Autodesk Fusion 360 part; units mm, degrees
sketch "Sketch1" plane through (0, 0, 0) normal (0, 1, 0) x (1, 0, 0)
  line L0 (20, -20) -> (-20, -20)
  line L1 (-20, -20) -> (-20, 20)
  line L2 (-20, 20) -> (20, 20)
  line L3 (20, 20) -> (20, -20)
  line L4 (20, -20) -> (-20, 20) construction
  line L5 (-20, -20) -> (20, 20) construction
  line L6 (-20, 4) -> (-15, 4)
  line L7 (-15, 4) -> (-15, -4)
  line L8 (-15, -4) -> (-20, -4)
  line L9 (-20, -4) -> (-20, 4)
  line L10 (-4, 20) -> (4, 20)
  line L11 (4, 20) -> (4, 15)
  line L12 (4, 15) -> (-4, 15)
  line L13 (-4, 15) -> (-4, 20)
  line L14 (20, 4) -> (15, 4)
  line L15 (15, 4) -> (15, -4)
  line L16 (15, -4) -> (20, -4)
  line L17 (20, -4) -> (20, 4)
  line L18 (-4, -20) -> (4, -20)
  line L19 (4, -20) -> (4, -15)
  line L20 (4, -15) -> (-4, -15)
  line L21 (-4, -15) -> (-4, -20)
  dimension "d1" = 40
  dimension "d2" = 40
  dimension "d3" = 5
  dimension "d4" = 8
  dimension "d5" = 16
  dimension "d6" = 5
  dimension "d7" = 16
  dimension "d8" = 8
  dimension "d9" = 5
  dimension "d10" = 5
  dimension "d11" = 8
  dimension "d12" = 8
  dimension "d13" = 16
  dimension "d14" = 16
extrude "Extrude1" add sketch "Sketch1" against normal blind 3 contours L0 L1 L2 L3 L6 L7 L8 L11 L12 L13 L14 L15 L16 L19 L20 L21
extrude "Extrude2" add sketch "Sketch1" against normal blind 8 contours L0 L18 L19 L20 L21 | L3 L14 L15 L16 L17 | L1 L6 L7 L8 L9 | L2 L10 L11 L12 L13
hole "Hole1" at (0, 0, 0) direction (0, -1, 0) diameter 9 depth 30 tip angle 118
fillet "Fillet1" radius 4 4 edges at (20, -1.5, -20) (-20, -1.5, -20) (20, -1.5, 20) (-20, -1.5, 20)
sketch "Sketch2" plane through (0, 0, 0) normal (0, 1, 0) x (1, 0, 0)
  line L0 (21, 21) -> (-21, 21)
  line L1 (-21, 21) -> (-21, -21)
  line L2 (-21, -21) -> (21, -21)
  line L3 (21, -21) -> (21, 21)
  line L4 (21, 21) -> (-21, -21) construction
  line L5 (-21, 21) -> (21, -21) construction
  dimension "d24" = 42
  dimension "d25" = 42
extrude "Extrude3" add sketch "Sketch2" sketch "Sketch1" along normal blind 30 of sketch 2 contours L0 L1 L2 L3 L6 L7 L8 L11 L12 L13 L14 L15 L16 L19 L20 L21
sketch "Sketch3" plane through (0, 30, 0) normal (0, 1, 0) x (-1, 0, 0)
  line L0 (-21, 21) -> (-21, -21)
  line L1 (-21, -21) -> (21, -21)
  line L2 (21, -21) -> (21, 21)
  line L3 (21, 21) -> (-21, 21)
  circle A0 centre (41, 0) radius 7.5
  circle A1 centre (-41, 0) radius 7.5
  line L4 (-21, -21) -> (-44.9086, -6.401)
  line L5 (-21, 21) -> (-44.9086, 6.401)
  line L6 (21, 21) -> (44.9086, 6.401)
  line L7 (21, -21) -> (44.9086, -6.401)
  point P0 (41, 0)
  point P1 (-41, 0)
  dimension "d28" = 21
  dimension "d29" = 41
  dimension "d30" = 41
  dimension "d31" = 15
  dimension "d32" = 15
extrude "Extrude4" add sketch "Sketch3" against normal blind 5 contours L0 A1 L4 L5 | L2 A0 L6 L7 | A1 | A0
sketch "Sketch4" plane through (0, 0, 0) normal (0, -1, 0) x (1, 0, 0)
  circle A0 centre (0, 0) radius 4.5
  circle A1 centre (0, 0) radius 4.5
sketch "Sketch5" plane through (0, 0, 0) normal (0, 1, 0) x (-1, 0, 0)
sketch "Sketch6" plane through (0, 30, 0) normal (0, 1, 0) x (-1, 0, 0)
  circle A0 centre (0, 0) radius 4.5
hole "Hole2" at (0, 30, 0) direction (0, -1, 0) diameter 10 depth 90 tip angle 118 counterbore diameter 14 counterbore depth 26
hole "Hole3" at (-41, 30, 0) at (41, 30, 0) direction (0, -1, 0) diameter 4.234 depth 90 tip angle 118
fillet "Fillet2" radius 4 4 edges at (21, 12.5, -21) (-21, 12.5, -21) (-21, 12.5, 21) (21, 12.5, 21)
equation "d6 = d3"
equation "d7 = d5"
equation "d8 = d4"
equation "d9 = d3"
equation "d10 = d3"
equation "d11 = d4"
equation "d12 = d4"
equation "d13 = d7"
equation "d14 = d7"
Model file for the job. Use its own axes, mm. A direction names the side the tool comes from. Give positions to 0.01 mm unless a question says otherwise; leave off trailing zeros. Loops run counter-clockwise (first coordinate to the right, second up) from the corner with the lowest first, then second, coordinate; pieces in that order, holes last.
1) Flat gauge pins, fed straight in: pin 1 Ø5.5 at (y, z) = (-4.5, -17) entering from -X; pin 2 Ø9 at (y, z) = (-3, -4.5) entering from -X; pin 3 Ø5.5 at (x, y) = (-17, -5.5) entering from -Z. Where does each tip first touch, or does it go through?
2) Saw through at B-B (y = 15). Write the cut outline in (x, z), plus the area to 3 significant figures.
3) Saw through at A-A (z = 0). Count the separate pieces of the cut face and the enclosed holes in it, plus the area to 3 significant figures.
4) Saw through at D-D (y = -5). Write the cut outline in (x, z), plus the area to 3 significant figures.
5) Saw through at C-C (x = 0). Write the cut outline in (y, z), plus the area to 3 significant figures.
6) Wall check: line 1 (X direction, y = 26.8, z = 0); line 2 (X direction, y = 9.75, z = 0); line 3 (Y direction, x = 2, z = 9). Give the ranges that are in metal, low to high.
7) Pull direction X, two halves, no side cores. Call faces 1 (the flat face through (-18, -8, 0)), 2 (the flat face through (-20, -3, 0)), 3 (the flat face through (-5, 4, -2)): +X half, -X half, draft (parallel to the pull), parting line (faces both ways), or undercut.
8) Tool access for faces 4 (the cylindrical face through (2.681, 16.818, 6.466)), 5 (the cylindrical face through (18.859, -1.521, 18.797)), 6 (the flat face through (-17, -5, 4)), 7 (the flat face through (21, 12, 0)): list every direction of +Z, -Z, +X, -X, +Y, -Y with a clear straight run to the whole face (end or side of a thin tool).
Answer block:
1. pin 1: stops at x = -20
1. pin 2: stops at x = -21
1. pin 3: stops at z = -20
2. outline: (-21, -17) arc R4 ccw to (-17, -21) - (17, -21) arc R4 ccw to (21, -17) - (21, 17) arc R4 ccw to (17, 21) - (-17, 21) arc R4 ccw to (-21, 17) - close; hole circle Ø14 at (0, 0)
2. area: 1,600 mm2
3. separate pieces: 4
3. enclosed holes: 0
3. area: 1,230 mm2
4. outline: (-20, -4) - (-15, -4) - (-15, 4) - (-20, 4) - close; (-4, -20) - (4, -20) - (4, -15) - (-4, -15) - close; (-4, 15) - (4, 15) - (4, 20) - (-4, 20) - close; (15, -4) - (20, -4) - (20, 4) - (15, 4) - close
4. area: 160 mm2
5. outline: (-8, -20) - (0, -20) - (0, -21) - (30, -21) - (30, -7) - (4, -7) - (4, -5) - (-3, -5) - (-3, -15) - (-8, -15) - close; (-8, 15) - (-3, 15) - (-3, 5) - (4, 5) - (4, 7) - (30, 7) - (30, 21) - (0, 21) - (0, 20) - (-8, 20) - close
5. area: 996 mm2
6. line 1: x = -48.5 to -43.12, -38.88 to -7, 7 to 38.88, 43.12 to 48.5
6. line 2: x = -21 to -7, 7 to 21
6. line 3: y = -3 to 30
7. face 1: draft
7. face 2: -X half
7. face 3: undercut
8. face 4: +Y
8. face 5: +Z, +X, -Y
8. face 6: +Z, +X, -X, -Y
8. face 7: +Z, -Z, +X, -Y
